Study the drawing (mm; zero at the part's minimum x, y, z) and answer. Give positions to 0.01 mm unless a question says otherwise; leave off trailing zeros. Order: outer loops, then holes, each group sorted by start corner. A loop starts at its lowest first (then second) coordinate and runs counter-clockwise, first axis right, second up.
Item 1: A cutting plane is placed at D-D (y = 10). Write down the section's boundary in (x, z), plus the area to 3 significant figures.
Item 2: A cutting plane is placed at B-B (x = 9.5). Write down the section's boundary in (y, z).
Item 3: A cutting plane is placed at A-A (z = 13.25). Write down the section's boundary in (x, y) (1 decimal), plus the area to 3 significant figures.
Item 4: The mould has two halves that part along Z. Classify the marked faces 1 and 2: +Z half, -Z half, draft (parallel to the pull), parting line (faces both ways), or undercut.
Item 5: Find the intervals of material crossed by line 1 along Y through (x, z) = (11, 12.5); line 2 along X through (y, z) = (13.5, 12) (1 decimal); line 3 along Y through (x, z) = (45, 9), in increasing order.
Item 6: A cutting plane is placed at C-C (y = 15.25). Write down the section's boundary in (x, z).
Item 7: Given pin 1 Ø10 at (x, y) = (34, 19.5) entering from +Z; pin 2 Ø5 at (x, z) = (6.5, 18) entering from +Y; pin 3 Ø1 at (x, y) = (33, 7) entering from +Z, each flat-ended and moving along its own axis, determine where each tip first touches the part or whether it passes through.
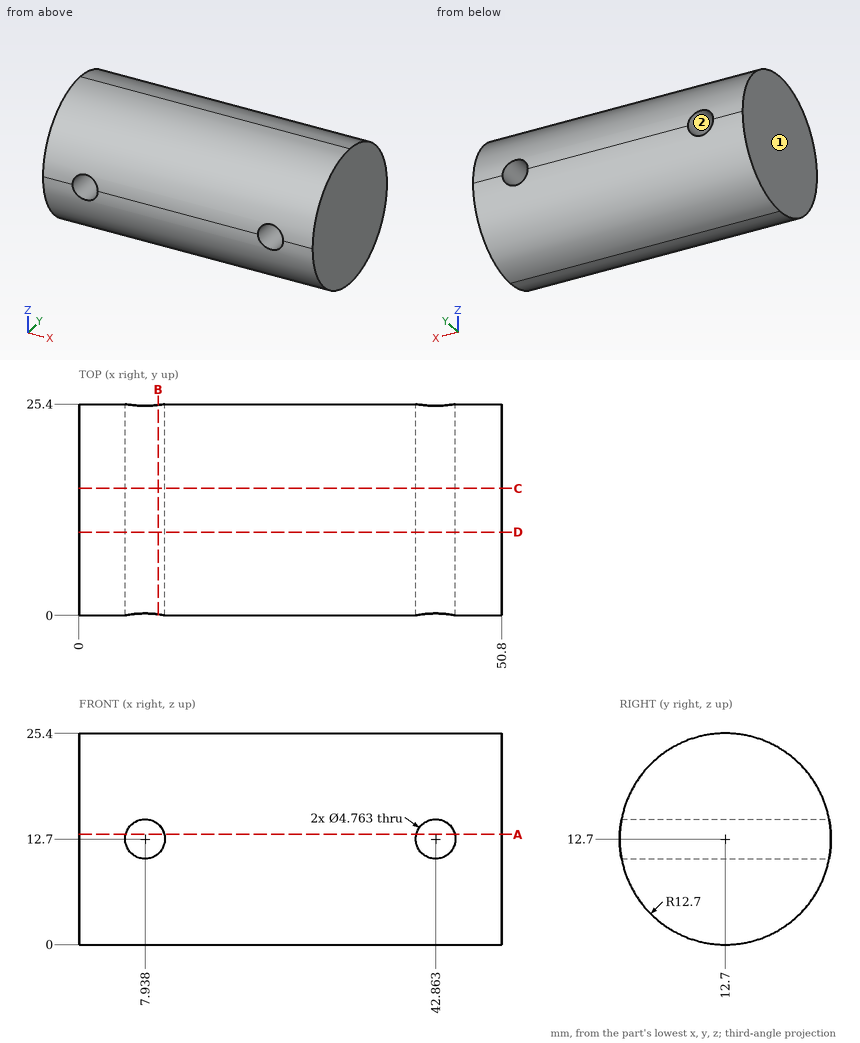
Response values:
1. outline: (0, 0.29) - (50.8, 0.29) - (50.8, 25.11) - (0, 25.11) - close; hole circle Ø4.76 at (7.94, 12.7); hole circle Ø4.76 at (42.86, 12.7)
1. area: 1,230 mm2
2. outline: (0.13, 10.9) arc R12.7 ccw to (25.27, 10.9) - close; (0.13, 14.5) - (25.27, 14.5) arc R12.7 ccw to start
3. outline: (0, 0) - (5.6, 0) - (5.6, 25.4) - (0, 25.4) - close; (10.3, 0) - (40.5, 0) - (40.5, 25.4) - (10.3, 25.4) - close; (45.2, 0) - (50.8, 0) - (50.8, 25.4) - (45.2, 25.4) - close
3. area: 1,050 mm2
4. face 1: draft
4. face 2: undercut
5. line 1: y = 0 to 25.4
5. line 2: x = 0 to 5.7, 10.2 to 40.6, 45.1 to 50.8
5. line 3: y = 0.55 to 24.85
6. outline: (0, 0.26) - (50.8, 0.26) - (50.8, 25.14) - (0, 25.14) - close; hole circle Ø4.76 at (7.94, 12.7); hole circle Ø4.76 at (42.86, 12.7)
7. pin 1: stops at z = 25.27
7. pin 2: stops at y = 25.09
7. pin 3: stops at z = 24.29
